Read the model definition and answer for the solid it produces. Units are mm, in the model's axes. Coordinates: 2 decimals unless noted, no trailing zeros. Write each loop counter-clockwise with the first axis right and the second up, starting at its lowest first coordinate (ties: lowest second). Pieces come first, ordered by that corner, then holes. Notation, with made-up numbers: (-22, 36) -> (15, 36) arc R28 cw to (15, 63) -> close; hole circle Ø1 at (80, -34). An arc over 180 degrees is marked (long way). Return JSON: item names as keys, results as strings.
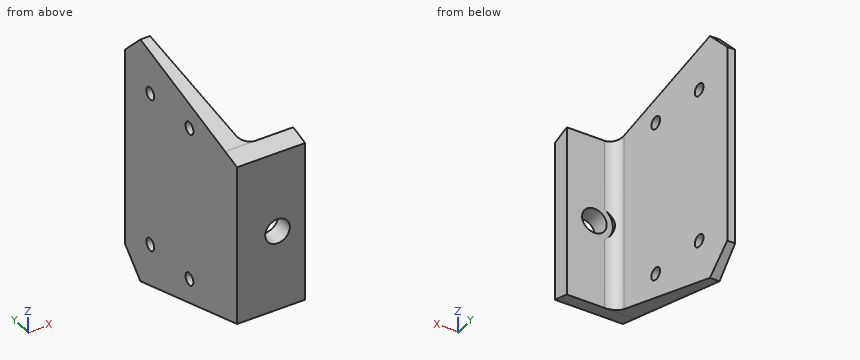
from build123d import *

# Parameters (mm, degrees)
SKETCH2_R               = 3.175
BOSS_EXTRUDE1_DEPTH     = 9.652
BOSS_EXTRUDE2_DEPTH     = 35.052
CUT_EXTRUDE1_DEPTH      = 117.316470579
CUT_EXTRUDE1_DEPTH_BACK = 117.316470579
FILLET1_R               = 6.35
SKETCH5_R               = 6.35
CUT_EXTRUDE3_DEPTH      = 109.937280598
CUT_EXTRUDE3_DEPTH_BACK = 109.937280598
SKETCH6_R               = 9.525
CUT_EXTRUDE4_DEPTH      = 109.937280598


with BuildPart() as part:
    # Sketch2 → Boss-Extrude1 (new body)
    with BuildSketch(Plane(origin=(0, 0, 0), x_dir=(0, 0, -1), z_dir=(1, 0, 0))):
        Polygon((0, 9.652), (43.903628026, 9.652), (63.5, 78.2912287), (50.8592287, 90.932), (0, 90.932), align=None)
        with Locations((39.624, 38.608)):
            Circle(SKETCH2_R, mode=Mode.SUBTRACT)
        with Locations((39.624, 70.358)):
            Circle(SKETCH2_R, mode=Mode.SUBTRACT)
        Polygon((-43.903628026, 9.652), (0, 9.652), (0, 90.932), (-50.8592287, 90.932), (-63.5, 78.2912287), align=None)
        with Locations((-39.624, 38.608)):
            Circle(SKETCH2_R, mode=Mode.SUBTRACT)
        with Locations((-39.624, 70.358)):
            Circle(SKETCH2_R, mode=Mode.SUBTRACT)
        Polygon((-41.148, 0), (0, 0), (0, 9.652), (-43.903628026, 9.652), align=None)
        Polygon((0, 0), (41.148, 0), (43.903628026, 9.652), (0, 9.652), align=None)
    extrude(amount=BOSS_EXTRUDE1_DEPTH)

    # Sketch2_6 → Boss-Extrude2 (add)
    with BuildSketch(Plane(origin=(0, 0, 0), x_dir=(0, 0, -1), z_dir=(1, 0, 0))):
        Polygon((-41.148, 0), (0, 0), (0, 9.652), (-43.903628026, 9.652), align=None)
        Polygon((0, 0), (41.148, 0), (43.903628026, 9.652), (0, 9.652), align=None)
    extrude(amount=BOSS_EXTRUDE2_DEPTH)

    # Sketch4 → Cut-Extrude1 (cut, two sides)
    with BuildSketch(Plane.XY) as cut_extrude1_sk:
        Polygon((9.652, 9.652), (4.064, 90.932), (9.652, 90.932), align=None)
    extrude(amount=CUT_EXTRUDE1_DEPTH, mode=Mode.SUBTRACT)
    extrude(cut_extrude1_sk.sketch, amount=-CUT_EXTRUDE1_DEPTH_BACK, mode=Mode.SUBTRACT)

    # Fillet1
    fillet1_edges = [part.edges().sort_by_distance(p)[0] for p in [
        (9.652, 9.652, 0),
    ]]
    fillet(fillet1_edges, radius=FILLET1_R)

    # Sketch5 → Cut-Extrude3 (cut, two sides)
    with BuildSketch(Plane(origin=(0, 9.652, 0), x_dir=(1, 0, 0), z_dir=(0, 1, 0))) as cut_extrude3_sk:
        with Locations(Location((20.828, 0, 0), (0, 0, 270))):
            Circle(SKETCH5_R)
    extrude(amount=CUT_EXTRUDE3_DEPTH, mode=Mode.SUBTRACT)
    extrude(cut_extrude3_sk.sketch, amount=-CUT_EXTRUDE3_DEPTH_BACK, mode=Mode.SUBTRACT)

    # Sketch6 → Cut-Extrude4 (cut, through all)
    with BuildSketch(Plane(origin=(0, 9.652, 0), x_dir=(1, 0, 0), z_dir=(0, 1, 0))):
        with Locations((20.828, 0)):
            Circle(SKETCH6_R)
    extrude(amount=CUT_EXTRUDE4_DEPTH, mode=Mode.SUBTRACT)


solid = part.part
1. The part is cut by section C-C (x = 31). Determine the outline of the cut face in (y, z).
Taken from the geometry:
{"outline": "(0, -41.15) -> (9.65, -43.9) -> (9.65, 43.9) -> (0, 41.15) -> close"}
2. The part is cut by section B-B (x = 24). Determine the outline of the cut face in (y, z), then the cut area to 3 significant figures.
Taken from the geometry:
{"outline": "(0, -41.15) -> (9.65, -43.9) -> (9.65, -5.5) -> (0, -5.5) -> close; (0, 5.5) -> (9.65, 5.5) -> (9.65, 43.9) -> (0, 41.15) -> close", "area": "715 mm2"}
3. The part is cut by section A-A (z = 0). Determine the outline of the cut face in (x, y).
Taken from the geometry:
{"outline": "(0, 0) -> (14.48, 0) -> (14.48, 9.65) -> (11.3, 9.65) -> (11.3, 11.31) arc R6.35 cw to (9.25, 15.57) -> (4.06, 90.93) -> (0, 90.93) -> close; (27.18, 0) -> (35.05, 0) -> (35.05, 9.65) -> (27.18, 9.65) -> close"}
4. Consider L1, parallel to Y at x = 26.5, z = -6.5; L2, parallel to X at y = 74, z = 55.5; L3, parallel to Y at x = 11, z = 2.5. Determine where each line is inside the solid, lowest interval first.
Taken from the geometry:
{"L1": "y = 0 to 9.65", "L2": "x = 0 to 5.23", "L3": "y = 0 to 11.6"}
5. The part is cut by section D-D (y = 50). Determine the outline of the cut face in (x, z).
Taken from the geometry:
{"outline": "(0, -55.42) -> (6.88, -55.42) -> (6.88, 55.42) -> (0, 55.42) -> close"}
6. Flat-ended cylindrical pins translate along their axes: pin 1 Ø7.5 at (y, z) = (38.608, -39.624) entering from +X; pin 2 Ø3 at (x, y) = (6, 59) entering from -Z; pin 3 Ø2 at (y, z) = (20, 36.5) entering from +X. Find the tip coordinate at first contact, or state that the pin passes through.
Taken from the geometry:
{"pin 1": "stops at x = 7.92", "pin 2": "stops at z = -58.42", "pin 3": "stops at x = 9.01"}
